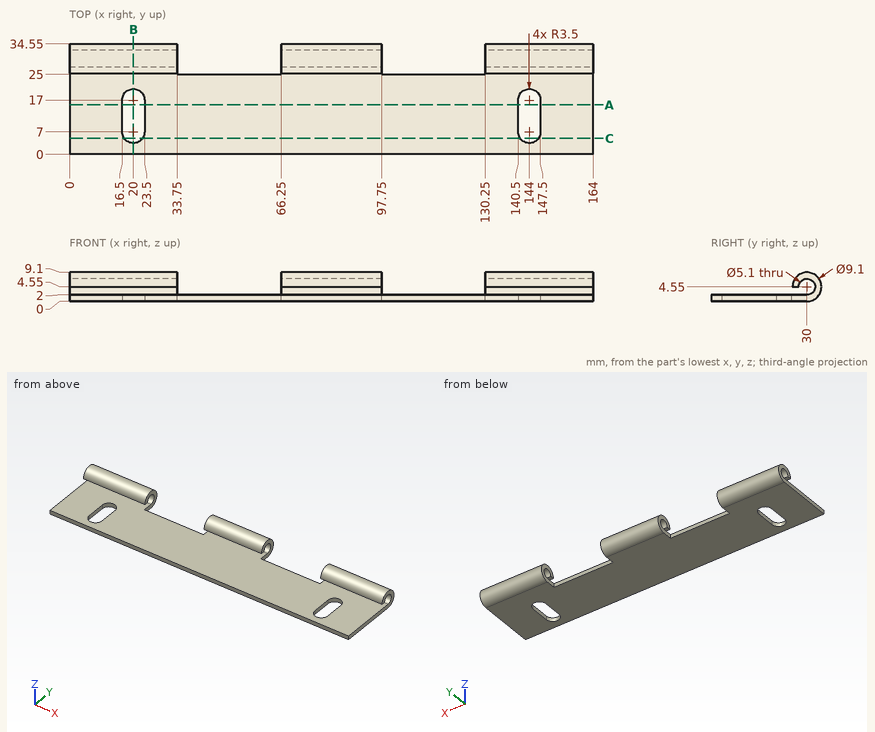
Input: dimensioned drawing with shaded views. Units: mm. Origin: part minimum x, y, z. Round coordinates to 2 decimals unless told otherwise and drop trailing zeros. Loops run counter-clockwise (first coordinate to the right, second up) from the corner with the lowest first, then second, coordinate; pieces in that order, holes last. Notation, with made-up numbers: M 57.5,20.25 L 73.5,20.25 A14 ccw 73.5,37.25 Z; hole C -8,64.25 d1. An arc over 180 degrees is marked long. One line per question, with ' | ' between items.
(1) Material intervals for line 1 along X through (y, z) = (27, 6.5); line 2 along Z through (x, y) = (150, 30); line 3 along X through (y, z) = (11.5, 1.5), sorted ascending. Write a range as from..to.
Check result:
line 1: x = 0..33.75, 66.25..97.75, 130.25..164 | line 2: z = 0..2, 7.1..9.1 | line 3: x = 0..16.5, 23.5..140.5, 147.5..164
(2) Cut plane B-B on x = 20. Return the cut outline in (y, z).
Check result:
outline: M 0,0 L 3.5,0 L 3.5,2 L 0,2 Z; M 20.5,0 L 30,0 A4.55 ccw long 25.45,4.55 L 27.45,4.55 A2.55 cw long 30,2 L 20.5,2 Z
(3) Contact query for flat-ended pins moving along their axis: P1, Ø1, axis at x = 47.5, y = 21, coming from the +Z side; P2, Ø2, axis at x = 46.5, z = 1.5, coming from the +Y side; P3, Ø1.5, axis at x = 84, z = 5.5, coming from the -Y side. Output: stop coordinate, or through.
Check result:
P1: stops at z = 2 | P2: stops at y = 25 | P3: stops at y = 25.45
(4) Cut plane C-C on y = 5. Return the cut outline in (x, z), plus the area to 3 significant figures.
Check result:
outline: M 0,0 L 17.13,0 L 17.13,2 L 0,2 Z; M 22.87,0 L 141.13,0 L 141.13,2 L 22.87,2 Z; M 146.87,0 L 164,0 L 164,2 L 146.87,2 Z | area: 305 mm2
(5) Cut plane A-A on y = 15.5. Return the cut outline in (x, z), plus the area to 3 significant figures.
Check result:
outline: M 0,0 L 16.5,0 L 16.5,2 L 0,2 Z; M 23.5,0 L 140.5,0 L 140.5,2 L 23.5,2 Z; M 147.5,0 L 164,0 L 164,2 L 147.5,2 Z | area: 300 mm2
